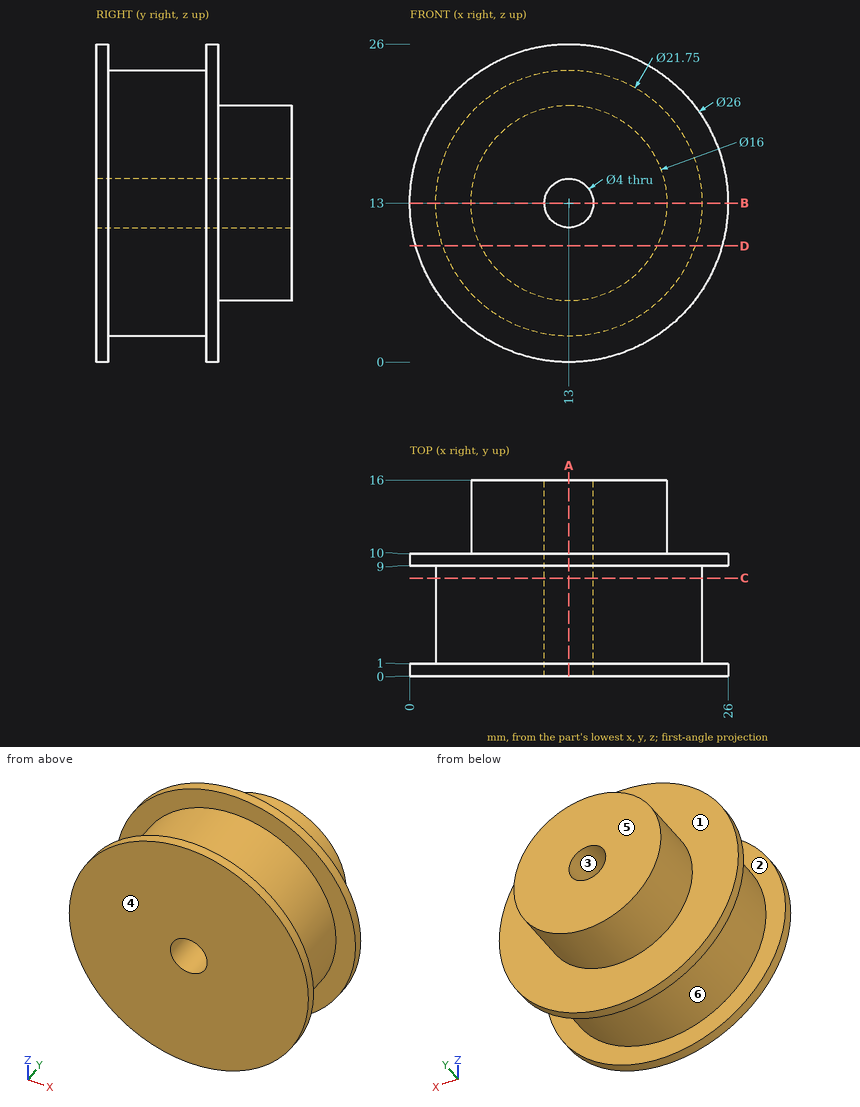
The drawing under review shows one solid part. Ordinate dimensions are in mm from its lowest x, y, z. A direction names the side the tool comes from. Give positions to 0.01 mm unless a question says otherwise; leave off trailing zeros. Write each loop counter-clockwise with the first axis right and the second up, starting at its lowest first coordinate (ties: lowest second). Pieces come first, ordered by that corner, then holes. Notation, with made-up numbers: (1, 40) -> (51, 40) arc R29 ccw to (51, 70) -> close; hole circle Ø7 at (-22, 25.25). An arc over 180 degrees is marked (long way). Use CSV: the item, a comma, the result in double quotes.
Q1. Take a section at A-A, the plane x = 13. Write out the cut boundary in (y, z) (3 decimals), then the cut area to 3 significant figures.
Conclusion:
outline,"(0, 0) -> (1, 0) -> (1, 2.125) -> (9, 2.125) -> (9, 0) -> (10, 0) -> (10, 5) -> (16, 5) -> (16, 11) -> (0, 11) -> close; (0, 15) -> (16, 15) -> (16, 21) -> (10, 21) -> (10, 26) -> (9, 26) -> (9, 23.875) -> (1, 23.875) -> (1, 26) -> (0, 26) -> close"
area,"258 mm2"
Q2. Tool access review of the marked faces 1, 2 and 3: name each direction out of +Z, -Z, +X, -X, +Y, -Y from which nothing blocks a thin tool from reaching the whole face with its end or side.
Conclusion:
face 1,"+Y"
face 2,"none"
face 3,"+Y, -Y"
Q3. To check wall thickness, follow probe 1 along X at (y, z) = (5.75, 13) (3 decimals); probe 2 along Y at (x, z) = (24, 6.75); probe 3 along X at (y, z) = (12, 13). State the ranges of each line that lie inside material, in increasing order. Write a range as [from, to].
Conclusion:
probe 1,"[2.125, 11], [15, 23.875]"
probe 2,"[0, 1], [9, 10]"
probe 3,"[5, 11], [15, 21]"
Q4. Take a section at B-B, the plane z = 13. Write out the cut boundary in (x, y) (3 decimals).
Conclusion:
outline,"(0, 0) -> (11, 0) -> (11, 16) -> (5, 16) -> (5, 10) -> (0, 10) -> (0, 9) -> (2.125, 9) -> (2.125, 1) -> (0, 1) -> close; (15, 0) -> (26, 0) -> (26, 1) -> (23.875, 1) -> (23.875, 9) -> (26, 9) -> (26, 10) -> (21, 10) -> (21, 16) -> (15, 16) -> close"
Q5. Take a section at D-D, the plane z = 9.5. Write out the cut boundary in (x, y).
Conclusion:
outline,"(0.48, 0) -> (25.52, 0) -> (25.52, 1) -> (23.3, 1) -> (23.3, 9) -> (25.52, 9) -> (25.52, 10) -> (20.19, 10) -> (20.19, 16) -> (5.81, 16) -> (5.81, 10) -> (0.48, 10) -> (0.48, 9) -> (2.7, 9) -> (2.7, 1) -> (0.48, 1) -> close"
Q6. Mouldability with a two-part tool opening along Y and no side actions: class the marked faces 4, 5 and 6 as pulls with the +Y half, pulls with the -Y half, needs draft (parallel to the pull), parting line crosses it, or undercut.
Conclusion:
face 4,"pulls with the -Y half"
face 5,"pulls with the +Y half"
face 6,"undercut"
Q7. Take a section at C-C, the plane y = 8. Write out the cut boundary in (x, z) (3 decimals), then the cut area to 3 significant figures.
Conclusion:
outline,"circle Ø21.75 at (13, 13); hole circle Ø4 at (13, 13)"
area,"359 mm2"
Q8. For P1, Ø3, axis at y = 7, z = 11.5, coming from the +X side (3 decimals); P2, Ø1, axis at y = 12.5, z = 18.5, coming from the -X side (3 decimals); P3, Ø2, axis at y = 7, z = 7, coming from the -X side, all flat-tipped, find the tip position at first contact; note any pin that passes through.
Conclusion:
P1,"x = 23.875"
P2,"x = 6.755"
P3,"x = 3.34"
